Can you work these out from the model? Positions are in its coordinate system, mm. Face numbers are marked on the shaded views. A direction names the side the tool comes from. Coordinates: 2 decimals unless noted, no trailing zeros. Order: outer loops, then holes, each group sorted by start corner. A loop starts at its lowest first (then second) coordinate and runs counter-clockwise, first axis right, second up. Notation, with made-up numbers: M -2.5,-21 L 20.5,-21 A25 ccw 20.5,13 Z; hole C -11,13 d1. An arc over 180 degrees is marked long. Answer as CSV lines item,"result". Start each with the question number.
1. If we section it at A-A (x = 31): List the corners of the cut face in (y, z) for me, plus the area to 4 significant figures.
2. On a 3-axis mill with a long thin cutter (end or side, diameter ignored), from which of +Z, -Z, +X, -X, +Y, -Y can I reach the whole of each face in a straight line? I mean the marked faces 3 and 4. Say none if no direction works.
3. If we mould it in two halves opening along Z, with no side actions, what happens to the marked faces 1 and 2? For each: released by +Z, released by -Z, zero draft, split by the parting line, or undercut.
4. I need wall thicknesses on line 1 along X through (y, z) = (2.25, 6); line 2 along Y through (x, z) = (-31, -1.5); line 3 along Z through (x, y) = (4, -2.5) (3 decimals). Which ranges of each line are inside material? Lowest first, please. Write a range as from..to.
5. If we section it at B-B (x = -35.5): List the corners of the cut face in (y, z) for me, plus the area to 3 significant figures.
6. Will these pins go through, and if not, where does the flat tip stop? pin 1 (1.5 mm diameter, centred on y = 2.5, z = -0.5, fed in from -X); pin 2 (0.7 mm diameter, centred on y = -0.5, z = -0.5, fed in from -X); pin 3 (6 mm diameter, centred on x = 23.5, z = -1.5, fed in from +Y).
```python
from build123d import *

# Parameters (mm, degrees)
SKETCH2_W                   = 95
SKETCH2_H                   = 15
BOSS_EXTRUDE1_DEPTH         = 3.25
CAVITY1_START               = -2.5
CAVITY1_DEPTH               = 2.5
CAVITY1_START_2             = -1.5
CAVITY1_2_DEPTH             = 4.75
CAVITY1_3_DEPTH             = 1.5
CUT_EXTRUDE1_START          = -5.75
CUT_EXTRUDE1_DEPTH          = 5.75
CUT_EXTRUDE2_START          = -1
CUT_EXTRUDE2_DEPTH          = 1
F_41_0_096_DIAMETER_HOLE1_D = 2.4384
CUT_EXTRUDE4_DEPTH          = 2
CAVITY2_START               = -3.25
CAVITY2_DEPTH               = 6.5
CAVITY2_START_2             = 0.75
CAVITY2_2_DEPTH             = 2.5
SKETCH12_W                  = 22.7
SKETCH12_H                  = 12.2
SKETCH12_W_2                = 22.5
SKETCH12_H_2                = 12
CUT_EXTRUDE6_DEPTH          = 2.5
CUT_EXTRUDE7_START          = -4
CUT_EXTRUDE7_DEPTH          = 4
SKETCH15_W                  = 8.5
SKETCH15_H                  = 4.25
SKETCH15_W_2                = 5
SKETCH15_H_2                = 3.25
CUT_EXTRUDE8_DEPTH          = 1.125


# Read off the part's stored shape, not the designer's step: Cavity1, Cavity2
with BuildPart() as part:
    # Sketch2 → Boss-Extrude1 (new, symmetric)
    with BuildSketch(Plane(origin=(0, 0, 0), x_dir=(1, 0, 0), z_dir=(0, 1, 0))):
        Rectangle(SKETCH2_W, SKETCH2_H)
    extrude(amount=BOSS_EXTRUDE1_DEPTH, both=True)

    # Cavity1 outline → Cavity1 (cut)
    with BuildSketch(Plane(origin=(0, 0, 0), x_dir=(1, 0, 0), z_dir=(0, 1, 0)).offset(CAVITY1_START)):
        with BuildLine():
            ThreePointArc((-47.5, 2.875), (-44.625, 0), (-47.5, -2.875))
            Line((-47.5, -2.875), (-47.5, -3.425))
            ThreePointArc((-47.5, -3.425), (-44.075, 0), (-47.5, 3.425))
            Line((-47.5, 3.425), (-47.5, 2.875))
        make_face()
        with BuildLine():
            Line((-47.5, 6.25), (-47.5, 4.5))
            ThreePointArc((-47.5, 4.5), (-43, 0), (-47.5, -4.5))
            Line((-47.5, -4.5), (-47.5, -6.25))
            ThreePointArc((-47.5, -6.25), (-45.523576462, -5.929270613), (-43.75, -5))
            Line((-43.75, -5), (-30.438820488, -2.75))
            ThreePointArc((-30.438820488, -2.75), (-28.114646288, 0), (-30.438820488, 2.75))
            Line((-30.438820488, 2.75), (-43.75, 5))
            ThreePointArc((-43.75, 5), (-45.523576462, 5.929270613), (-47.5, 6.25))
        make_face()
    extrude(amount=CAVITY1_DEPTH, mode=Mode.SUBTRACT)

    # Cavity1 2 outline → Cavity1 2 (cut)
    with BuildSketch(Plane(origin=(0, 0, 0), x_dir=(1, 0, 0), z_dir=(0, 1, 0)).offset(CAVITY1_START_2)):
        with BuildLine():
            ThreePointArc((-47.5, 3), (-44.5, 0), (-47.5, -3))
            Line((-47.5, -3), (-47.5, -4.5))
            ThreePointArc((-47.5, -4.5), (-43, 0), (-47.5, 4.5))
            Line((-47.5, 4.5), (-47.5, 3))
        make_face()
    extrude(amount=CAVITY1_2_DEPTH, mode=Mode.SUBTRACT)

    # Cavity1 3 outline → Cavity1 3 (cut)
    with BuildSketch(Plane(origin=(0, 0, 0), x_dir=(1, 0, 0), z_dir=(0, 1, 0)).offset(CAVITY1_START_2)):
        with BuildLine():
            Line((-47.5, 2.875), (-47.5, 1.5))
            ThreePointArc((-47.5, 1.5), (-46, 0), (-47.5, -1.5))
            Line((-47.5, -1.5), (-47.5, -2.875))
            ThreePointArc((-47.5, -2.875), (-44.625, 0), (-47.5, 2.875))
        make_face()
    extrude(amount=CAVITY1_3_DEPTH, mode=Mode.SUBTRACT)

    # Sketch4 → Cut-Extrude1 (cut)
    with BuildSketch(Plane(origin=(0, 3.25, 0), x_dir=(1, 0, 0), z_dir=(0, 1, 0)).offset(CUT_EXTRUDE1_START)):
        with BuildLine():
            Line((-47.5, 3), (-47.5, -3))
            ThreePointArc((-47.5, -3), (-44.5, 0), (-47.5, 3))
        make_face()
    extrude(amount=CUT_EXTRUDE1_DEPTH, mode=Mode.SUBTRACT)

    # Sketch6 → Cut-Extrude2 (cut)
    with BuildSketch(Plane(origin=(0, -1.5, 0), x_dir=(1, 0, 0), z_dir=(0, 1, 0)).offset(CUT_EXTRUDE2_START)):
        with BuildLine():
            Line((-47.5, 4.5), (-47.5, 3.425))
            ThreePointArc((-47.5, 3.425), (-44.075, 0), (-47.5, -3.425))
            Line((-47.5, -3.425), (-47.5, -4.5))
            ThreePointArc((-47.5, -4.5), (-43, 0), (-47.5, 4.5))
        make_face()
    extrude(amount=CUT_EXTRUDE2_DEPTH, mode=Mode.SUBTRACT)

    # #41 (0.096) Diameter Hole1 (through all)
    with Locations(Plane(origin=(0, -3.25, 0), x_dir=(-1, 0, 0), z_dir=(0, -1, 0))):
        with Locations((-44, 0), (-16.7, 0)):
            Hole(F_41_0_096_DIAMETER_HOLE1_D / 2)

    # Sketch10 → Cut-Extrude4 (cut)
    with BuildSketch(Plane.XZ.offset(3.25)):
        Polygon((46.5, -1.443375673), (46.5, 1.443375673), (44, 2.886751346), (41.5, 1.443375673), (41.5, -1.443375673), (44, -2.886751346), align=None)
        Polygon((16.7, 2.886751346), (14.2, 1.443375673), (14.2, -1.443375673), (16.7, -2.886751346), (19.2, -1.443375673), (19.2, 1.443375673), align=None)
    extrude(amount=-CUT_EXTRUDE4_DEPTH, mode=Mode.SUBTRACT)

    # Cavity2 outline → Cavity2 (cut)
    with BuildSketch(Plane(origin=(0, 0, 0), x_dir=(1, 0, 0), z_dir=(0, 1, 0)).offset(CAVITY2_START)):
        with BuildLine():
            ThreePointArc((30.267317748, -2.75), (41.6, 0), (30.267317748, 2.75))
            ThreePointArc((30.267317748, 2.75), (27.1, 0), (30.267317748, -2.75))
        make_face()
    extrude(amount=CAVITY2_DEPTH, mode=Mode.SUBTRACT)

    # Cavity2 2 outline → Cavity2 2 (cut)
    with BuildSketch(Plane(origin=(0, 0, 0), x_dir=(1, 0, 0), z_dir=(0, 1, 0)).offset(CAVITY2_START_2)):
        with BuildLine():
            Line((19.1, 6), (19.1, -6))
            Line((19.1, -6), (35.6, -6))
            ThreePointArc((35.6, -6), (32.477501001, -5.123475383), (30.267317748, -2.75))
            ThreePointArc((30.267317748, -2.75), (27.1, 0), (30.267317748, 2.75))
            ThreePointArc((30.267317748, 2.75), (32.477501001, 5.123475383), (35.6, 6))
            Line((35.6, 6), (19.1, 6))
        make_face()
        with BuildLine():
            ThreePointArc((41.5, -1.090871211), (39.4376277, -4.61222437), (35.6, -6))
            Line((35.6, -6), (41.6, -6))
            Line((41.6, -6), (41.6, 0))
            ThreePointArc((41.6, 0), (41.574947699, -0.547722558), (41.5, -1.090871211))
        make_face()
        with BuildLine():
            Line((41.6, 6), (35.6, 6))
            ThreePointArc((35.6, 6), (39.4376277, 4.612224369), (41.5, 1.090871211))
            ThreePointArc((41.5, 1.090871211), (41.574947699, 0.547722558), (41.6, 0))
            Line((41.6, 0), (41.6, 6))
        make_face()
    extrude(amount=CAVITY2_2_DEPTH, mode=Mode.SUBTRACT)

    # Sketch12 → Cut-Extrude6 (cut)
    with BuildSketch(Plane(origin=(0, 0.75, 0), x_dir=(1, 0, 0), z_dir=(0, 1, 0))):
        with Locations((30.35, 0)):
            Rectangle(SKETCH12_W, SKETCH12_H)
        with Locations((30.35, 0)):
            Rectangle(SKETCH12_W_2, SKETCH12_H_2, mode=Mode.SUBTRACT)
    extrude(amount=CUT_EXTRUDE6_DEPTH, mode=Mode.SUBTRACT)

    # Sketch13 → Cut-Extrude7 (cut)
    with BuildSketch(Plane(origin=(0, 0.75, 0), x_dir=(1, 0, 0), z_dir=(0, 1, 0)).offset(CUT_EXTRUDE7_START)):
        with BuildLine():
            ThreePointArc((30.211004889, -2.858099316), (41.7, 0), (30.211004889, 2.858099316))
            ThreePointArc((30.211004889, 2.858099316), (27, 0), (30.211004889, -2.858099316))
        make_face()
        with BuildLine():
            ThreePointArc((30.267317748, 2.75), (41.6, 0), (30.267317748, -2.75))
            ThreePointArc((30.267317748, -2.75), (27.1, 0), (30.267317748, 2.75))
        make_face(mode=Mode.SUBTRACT)
    extrude(amount=CUT_EXTRUDE7_DEPTH, mode=Mode.SUBTRACT)

    # Sketch15 → Cut-Extrude8 (cut, symmetric)
    with BuildSketch(Plane.XY):
        with Locations((3.75, -1.125)):
            Rectangle(SKETCH15_W, SKETCH15_H)
        with Locations((-3, -0.625)):
            Rectangle(SKETCH15_W_2, SKETCH15_H_2)
    extrude(amount=CUT_EXTRUDE8_DEPTH, both=True, mode=Mode.SUBTRACT)


solid = part.part
```
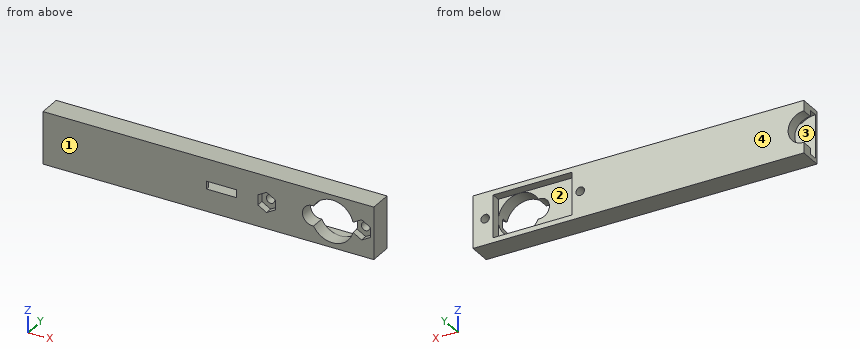
Solved:
1,outline,"M -3.25,-7.5 L 3.25,-7.5 L 3.25,-6.1 L 0.75,-6.1 L 0.75,-4.01 L -3.25,-4.01 Z; M -3.25,4.01 L 0.75,4.01 L 0.75,6.1 L 3.25,6.1 L 3.25,7.5 L -3.25,7.5 Z"
1,area,"34.95 mm²"
2,face 3,"-X"
2,face 4,"+Z, -Z, +X, -X, +Y"
3,face 1,"zero draft"
3,face 2,"undercut"
4,line 1,"-47.5..19, 41.7..47.5"
4,line 2,"-3.25..-2.5, 0..3.25"
4,line 3,"-7.5..-1.125, 1.125..7.5"
5,outline,"M -3.25,-7.5 L 3.25,-7.5 L 3.25,7.5 L -3.25,7.5 Z; hole M -2.5,-3.61 L 0,-3.61 L 0,3.61 L -2.5,3.61 Z"
5,area,"79.5 mm²"
6,pin 1,"x = -43.18"
6,pin 2,"x = -28.25"
6,pin 3,"y = 0.75"
